Here's how the part is built. I have some questions about the finished solid (model axes, mm). A direction names the side the tool comes from. Coordinates: 2 decimals unless noted, no trailing zeros. Write each loop counter-clockwise with the first axis right and the second up, starting at its lowest first coordinate (ties: lowest second). Pieces come first, ordered by that corner, then holes.
from build123d import *

# Parameters (mm, degrees)
F0_W     = 42
F0_H     = 42
F1_DEPTH = 42
F2_R     = 2
F3_DEPTH = 25
F4_R     = 1.5
F5_DEPTH = 16


with BuildPart() as f1:
    # F0 (on Top) → F1 (new body)
    with BuildSketch(Plane.XY):
        Rectangle(F0_W, F0_H)
    extrude(amount=F1_DEPTH)

    # F2 (on face) → F3 (join)
    with BuildSketch(Plane(origin=(0, 0, 0), x_dir=(1, 0, 0), z_dir=(0, 0, -1))):
        Circle(F2_R)
    extrude(amount=F3_DEPTH)

    # F4 (on face) → F5 (join)
    with BuildSketch(Plane(origin=(0, 0, 0), x_dir=(1, 0, 0), z_dir=(0, 0, -1))):
        with Locations((-15, 15)):
            Circle(F4_R)
        with Locations((15, 15)):
            Circle(F4_R)
        with Locations((15, -15)):
            Circle(F4_R)
        with Locations((-15, -15)):
            Circle(F4_R)
    extrude(amount=F5_DEPTH)


solid = f1.part
1. I want a section at A-A (z = -8.5). List the corners of the cut face in (x, y) for me, then the cut area to 3 significant figures.
2. For pin 1 Ø6 at (x, y) = (-8, 16) entering from -Z; pin 2 Ø2.5 at (x, y) = (-15.5, -14.5) entering from -Z; pin 3 Ø12 at (y, z) = (11.5, -10.5) entering from -X, each with a flat end and sliding along its axis, tell me the tip position at first contact or that it passes through.
3. I want a section at C-C (y = 0). List the corners of the cut face in (x, z) for me.
4. I want a section at B-B (x = 15). List the corners of the cut face in (y, z) for me.
5. On a 3-axis mill with a long thin cutter (end or side, diameter ignored), from which of +Z, -Z, +X, -X, +Y, -Y can I reach the whole of each face in a straight line? I mean faces 1 (the face through (-16.5, 14.93, -7.89)), 2 (the face through (0, 0, 42)). Say none if no direction works.
6. Thinking about a two-plate mould opening in Y: for faces 3 (the face through (0, -21, 21)), 4 (the face through (15, 15, -16)), 5 (the face through (13.5, -15.07, -7.89)), which applies, pulls with the +Y half, pulls with the -Y half, needs draft (parallel to the pull), parting line crosses it, or undercut?
7. If I drill on line 1 (Z direction, x = -3, y = -5); line 2 (X direction, y = 15.5, z = -11), over which ranges is the centre line in solid material (lowest first)?
Response values:
1. outline: circle Ø3 at (-15, -15); circle Ø3 at (-15, 15); circle Ø4 at (0, 0); circle Ø3 at (15, -15); circle Ø3 at (15, 15)
1. area: 40.8 mm2
2. pin 1: stops at z = 0
2. pin 2: stops at z = -16
2. pin 3: stops at x = -16.5
3. outline: (-21, 0) - (-2, 0) - (-2, -25) - (2, -25) - (2, 0) - (21, 0) - (21, 42) - (-21, 42) - close
4. outline: (-21, 0) - (-16.5, 0) - (-16.5, -16) - (-13.5, -16) - (-13.5, 0) - (13.5, 0) - (13.5, -16) - (16.5, -16) - (16.5, 0) - (21, 0) - (21, 42) - (-21, 42) - close
5. face 1: -Z
5. face 2: +Z, +X, -X, +Y, -Y
6. face 3: pulls with the -Y half
6. face 4: needs draft
6. face 5: undercut
7. line 1: z = 0 to 42
7. line 2: x = -16.41 to -13.59, 13.59 to 16.41
